For this review, take the finished solid that the model builds, in its own axes (mm). A direction names the side the tool comes from. Give positions to 0.01 mm unless a question says otherwise; leave off trailing zeros. Order: outer loops, then holes, each group sorted by start corner. A loop starts at its lowest first (then second) coordinate and runs counter-clockwise, first axis right, second up. Notation, with made-up numbers: (-3.75, 40) - (39.25, 40) arc R31 cw to (39.25, 74) - close; hole circle Ø2 at (50, 12). An arc over 180 degrees is marked (long way). Answer as a JSON object with one key per item and string values. Group by question number.
from build123d import *

# Parameters (mm, degrees)
SKETCH3_W           = 246
SKETCH3_H           = 154
SKETCH3_W_2         = 120
SKETCH3_H_2         = 50
BOSS_EXTRUDE1_DEPTH = 3
SKETCH4_R           = 2.54
CUT_EXTRUDE1_DEPTH  = 47.752


with BuildPart() as part:
    # Sketch3 → Boss-Extrude1 (new body)
    with BuildSketch(Plane.XY):
        with BuildLine():
            Line((-128.49, -145), (128.49, -145))
            ThreePointArc((128.49, -145), (140.164332957, -140.164332957), (145, -128.49))
            Line((145, -128.49), (145, 128.49))
            ThreePointArc((145, 128.49), (140.164332957, 140.164332957), (128.49, 145))
            Line((128.49, 145), (-128.49, 145))
            ThreePointArc((-128.49, 145), (-140.164332957, 140.164332957), (-145, 128.49))
            Line((-145, 128.49), (-145, -128.49))
            ThreePointArc((-145, -128.49), (-140.164332957, -140.164332957), (-128.49, -145))
        make_face()
        with Locations((0, -45.5)):
            Rectangle(SKETCH3_W, SKETCH3_H, mode=Mode.SUBTRACT)
        with BuildLine():
            Line((-38.77, 74.35), (-51.23, 74.35))
            ThreePointArc((-51.23, 74.35), (-51.449203102, 74.259203102), (-51.54, 74.04))
            Line((-51.54, 74.04), (-51.54, 68.96))
            ThreePointArc((-51.54, 68.96), (-51.449203102, 68.740796898), (-51.23, 68.65))
            Line((-51.23, 68.65), (-38.77, 68.65))
            ThreePointArc((-38.77, 68.65), (-38.550796898, 68.740796898), (-38.46, 68.96))
            Line((-38.46, 68.96), (-38.46, 74.04))
            ThreePointArc((-38.46, 74.04), (-38.550796898, 74.259203102), (-38.77, 74.35))
        make_face(mode=Mode.SUBTRACT)
        with Locations((50, 88.25)):
            Rectangle(SKETCH3_W_2, SKETCH3_H_2, mode=Mode.SUBTRACT)
        Polygon((-57.298294078, 105), (-63.649147039, 116), (-76.350852961, 116), (-82.701705922, 105), (-76.350852961, 94), (-63.649147039, 94), align=None, mode=Mode.SUBTRACT)
        Polygon((-84.030344885, 71.5), (-89.515172443, 81), (-100.484827557, 81), (-105.969655115, 71.5), (-100.484827557, 62), (-89.515172443, 62), align=None, mode=Mode.SUBTRACT)
    extrude(amount=-BOSS_EXTRUDE1_DEPTH)

    # Sketch4 → Cut-Extrude1 (cut)
    with BuildSketch(Plane.XY):
        with Locations((-133.604, 94.742)):
            Circle(SKETCH4_R)
        with Locations((-106.172, 134.62)):
            Circle(SKETCH4_R)
        with Locations((-133.604, -94.742)):
            Circle(SKETCH4_R)
        with Locations((-133.604, 0)):
            Circle(SKETCH4_R)
        with Locations((0, 134.62)):
            Circle(SKETCH4_R)
        with Locations((0, -134.62)):
            Circle(SKETCH4_R)
        with Locations((-106.172, -134.62)):
            Circle(SKETCH4_R)
        with Locations((106.172, -134.62)):
            Circle(SKETCH4_R)
        with Locations((133.604, 0)):
            Circle(SKETCH4_R)
        with Locations((133.604, -94.742)):
            Circle(SKETCH4_R)
        with Locations((106.172, 134.62)):
            Circle(SKETCH4_R)
        with Locations((133.604, 94.742)):
            Circle(SKETCH4_R)
    extrude(amount=-CUT_EXTRUDE1_DEPTH, mode=Mode.SUBTRACT)


solid = part.part
1) For line 1 (Y direction, x = -68, z = -2.6); line 2 (Y direction, x = -46.5, z = -0.95); line 3 (Y direction, x = 0, z = -0.6), list the stretches that pass through material, from the lowest coordinate up.
2) Consider section A-A (y = -76.5). Give the boundary of the cut face in (x, z).
3) Consider section C-C (x = -30). Give the boundary of the cut face in (y, z), plus the area to 3 significant figures.
4) For pin 1 (8 mm diameter, centred on x = 106.172, y = -134.62, fed in from +Z), flat-tipped, find the tip position at first contact; note if it passes through.
5) Consider section D-D (x = -94.5). Give the boundary of the cut face in (y, z).
6) For faces 5 (the face through (-60.52, 99.42, -1.48)), 6 (the face through (-2, 34, -3)), list the 3-axis set-ups (+Z, -Z, +X, -X, +Y, -Y) from which the entire face can be reached by the end or side of a thin tool; tool diameter is ignored.
7) Consider section B-B (x = 53.5). Give the boundary of the cut face in (y, z), plus the area to 3 significant figures.
8) Mouldability with a two-part tool opening along X and no side actions: class faces 1 (the face through (140.04, -140.29, -1.48)), 2 (the face through (-79.48, 110.58, -1.48)), 3 (the face through (-140.04, 140.29, -1.48)), 4 (the face through (-2, 34, 0)) as released by +X, released by -X, zero draft, split by the parting line, or undercut.
Result set:
{
 "1": {"line 1": "y = -145 to -122.5, 31.5 to 94, 116 to 145", "line 2": "y = -145 to -122.5, 31.5 to 68.65, 74.35 to 145", "line 3": "y = -145 to -137.16, -132.08 to -122.5, 31.5 to 63.25, 113.25 to 132.08, 137.16 to 145"},
 "2": {"outline": "(-145, -3) - (-123, -3) - (-123, 0) - (-145, 0) - close; (123, -3) - (145, -3) - (145, 0) - (123, 0) - close"},
 "3": {"outline": "(-145, -3) - (-122.5, -3) - (-122.5, 0) - (-145, 0) - close; (31.5, -3) - (145, -3) - (145, 0) - (31.5, 0) - close", "area": "408 mm2"},
 "4": {"pin 1": "stops at z = 0"},
 "5": {"outline": "(-145, -3) - (-122.5, -3) - (-122.5, 0) - (-145, 0) - close; (31.5, -3) - (62, -3) - (62, 0) - (31.5, 0) - close; (81, -3) - (145, -3) - (145, 0) - (81, 0) - close"},
 "6": {"face 5": "+Z, -Z", "face 6": "-Z, +X, -X, +Y, -Y"},
 "7": {"outline": "(-145, -3) - (-122.5, -3) - (-122.5, 0) - (-145, 0) - close; (31.5, -3) - (63.25, -3) - (63.25, 0) - (31.5, 0) - close; (113.25, -3) - (145, -3) - (145, 0) - (113.25, 0) - close", "area": "258 mm2"},
 "8": {"face 1": "released by +X", "face 2": "undercut", "face 3": "released by -X", "face 4": "zero draft"}
}
